```python
from build123d import *

# Parameters (mm, degrees)
SKETCH1_W           = 57.15
SKETCH1_H           = 101.6
BOSS_EXTRUDE1_DEPTH = 3.175
SKETCH2_W           = 6.35
SKETCH2_H           = 12.7
BOSS_EXTRUDE2_DEPTH = 3.175
LPATTERN1_COUNT     = 4
LPATTERN1_PITCH     = 25.4
SKETCH3_W           = 50.8
SKETCH3_H           = 15.875
BOSS_EXTRUDE3_DEPTH = 3.175
SKETCH4_W           = 19.05
SKETCH4_H           = 88.9
CUT_EXTRUDE1_DEPTH  = 3.175
FILLET1_R           = 6.35


with BuildPart() as part:
    # Sketch1 → Boss-Extrude1 (new body)
    with BuildSketch(Plane.XY):
        with Locations((28.575, -50.8)):
            Rectangle(SKETCH1_W, SKETCH1_H)
    extrude(amount=BOSS_EXTRUDE1_DEPTH)

    # Sketch2 → Boss-Extrude2 (add)
    with BuildSketch(Plane.XY.offset(3.175)):
        with Locations((60.325, -19.05)):
            Rectangle(SKETCH2_W, SKETCH2_H)
        with Locations((-3.175, -19.05)):
            Rectangle(SKETCH2_W, SKETCH2_H)
    boss_extrude2 = extrude(amount=-BOSS_EXTRUDE2_DEPTH)

    # LPattern1: Boss-Extrude2 ×4
    with Locations(*[(0, -i * LPATTERN1_PITCH, 0) for i in range(1, LPATTERN1_COUNT)]):
        add(boss_extrude2)

    # Sketch3 → Boss-Extrude3 (add)
    with BuildSketch(Plane.XY.offset(3.175)):
        with Locations((28.575, -109.5375)):
            Rectangle(SKETCH3_W, SKETCH3_H)
    extrude(amount=-BOSS_EXTRUDE3_DEPTH)

    # Sketch4 → Cut-Extrude1 (cut)
    with BuildSketch(Plane.XY.offset(3.175)):
        with Locations((15.875, -50.8)):
            Rectangle(SKETCH4_W, SKETCH4_H)
        with Locations((41.275, -50.8)):
            Rectangle(SKETCH4_W, SKETCH4_H)
    extrude(amount=-CUT_EXTRUDE1_DEPTH, mode=Mode.SUBTRACT)

    # Fillet1
    fillet1_edges = [part.edges().sort_by_distance(p)[0] for p in [
        (6.35, -95.25, 1.5875),
        (6.35, -6.35, 1.5875),
        (25.4, -6.35, 1.5875),
        (25.4, -95.25, 1.5875),
        (50.8, -6.35, 1.5875),
        (50.8, -95.25, 1.5875),
        (31.75, -95.25, 1.5875),
        (31.75, -6.35, 1.5875),
    ]]
    fillet(fillet1_edges, radius=FILLET1_R)


solid = part.part
```
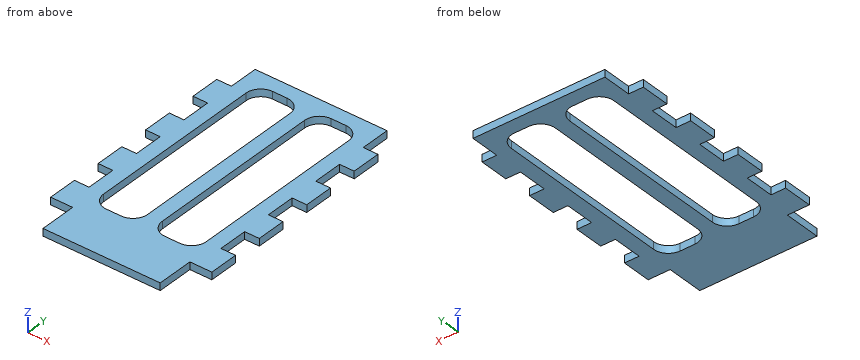
Read the model definition and answer for the solid it produces. Units are mm, in the model's axes. Coordinates: 2 decimals unless noted, no trailing zeros. Write each loop counter-clockwise with the first axis right and the second up, starting at its lowest first coordinate (ties: lowest second). Pieces come first, ordered by that corner, then holes. Notation, with made-up numbers: (28, 57) -> (66, 57) arc R16 cw to (66, 69) -> close; hole circle Ø11 at (-36.75, -25.75). An arc over 180 degrees is marked (long way). Answer as a JSON object with one key per item and string values.
Q1. The part is cut by section D-D on y = -109.5. Give the vertices of the cut face in (x, z) (3 decimals).
The answers:
{"outline": "(3.175, 0) -> (53.975, 0) -> (53.975, 3.175) -> (3.175, 3.175) -> close"}
Q2. The part is cut by section A-A on y = -70. Give the vertices of the cut face in (x, z) (3 decimals), then the cut area to 3 significant figures.
The answers:
{"outline": "(-6.35, 0) -> (6.35, 0) -> (6.35, 3.175) -> (-6.35, 3.175) -> close; (25.4, 0) -> (31.75, 0) -> (31.75, 3.175) -> (25.4, 3.175) -> close; (50.8, 0) -> (63.5, 0) -> (63.5, 3.175) -> (50.8, 3.175) -> close", "area": "101 mm2"}
Q3. Consider line 1 (X direction, y = -76.5, z = 2.2); line 2 (X direction, y = -23, z = 1.45); line 3 (Y direction, x = -3, z = 0.6). Determine where each line is inside the solid, lowest interval first. Write a range as [from, to].
The answers:
{"line 1": "x = [0, 6.35], [25.4, 31.75], [50.8, 57.15]", "line 2": "x = [-6.35, 6.35], [25.4, 31.75], [50.8, 63.5]", "line 3": "y = [-101.6, -88.9], [-76.2, -63.5], [-50.8, -38.1], [-25.4, -12.7]"}
Q4. The part is cut by section C-C on z = 0.6. Give the number of separate pieces and of enclosed holes in the cut face, then the cut area to 3 significant figures.
The answers:
{"separate pieces": "1", "enclosed holes": "2", "area": "3,940 mm2"}
Q5. Flat-ended cylindrical pins translate along their axes: pin 1 Ø1.6 at (x, z) = (61.5, 1.5) entering from +Y; pin 2 Ø1.5 at (y, z) = (-25.5, 1) entering from -X; pin 3 Ø1.6 at (y, z) = (-55, 1) entering from +X. Find the tip coordinate at first contact, or state that the pin passes through.
The answers:
{"pin 1": "stops at y = -12.7", "pin 2": "stops at x = -6.35", "pin 3": "stops at x = 57.15"}
Q6. The part is cut by section B-B on x = 34.5. Give the vertices of the cut face in (y, z) (3 decimals), then the cut area to 3 significant figures.
The answers:
{"outline": "(-117.475, 0) -> (-94.131, 0) -> (-94.131, 3.175) -> (-117.475, 3.175) -> close; (-7.469, 0) -> (0, 0) -> (0, 3.175) -> (-7.469, 3.175) -> close", "area": "97.8 mm2"}
